Print and shaded views of the part. All mm, measured from the part's lowest x, y and z. A direction names the side the tool comes from. Round coordinates to 2 decimals unless told otherwise and drop trailing zeros. Loops run counter-clockwise (first coordinate to the right, second up) from the corner with the lowest first, then second, coordinate; pieces in that order, holes last. Notation, with made-up numbers: (13, 18) -> (48, 18) arc R25 ccw to (48, 46) -> close; hole circle Ø4 at (-5, -24.75). An arc over 180 degrees is marked (long way). Use a Markdown table: item, result.
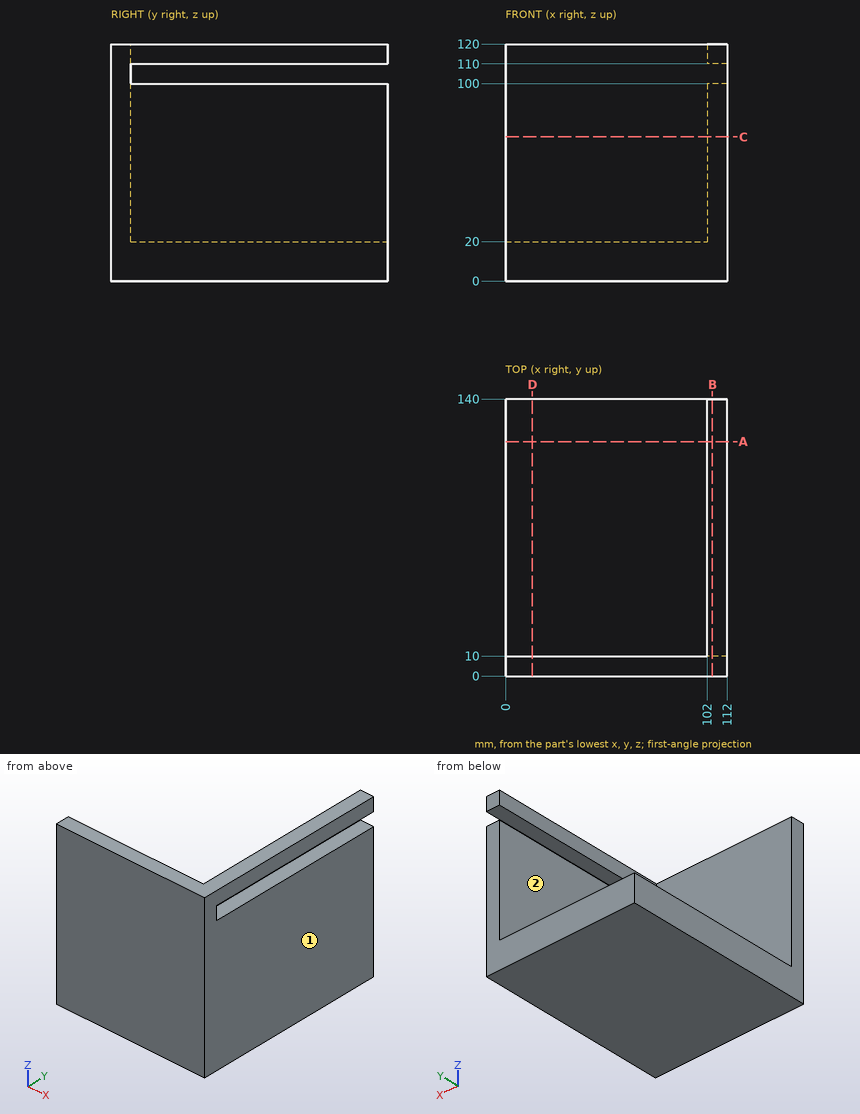
Q1. Tool access for the marked faces 1 and 2: list every direction of +Z, -Z, +X, -X, +Y, -Y with a clear straight run to the whole face (end or side of a thin tool).
Results list:
| item | result |
|---|---|
| face 1 | +Z, -Z, +X, +Y, -Y |
| face 2 | +Z, -X, +Y |
Q2. Flat gauge pins, fed straight in: pin 1 (5 mm diameter, centred on x = 85.5, z = 106, fed in from -Y); pin 2 (2 mm diameter, centred on x = 18, y = 107.5, fed in from +Z); pin 3 (10 mm diameter, centred on x = 65.5, z = 36.5, fed in from +Y); pin 4 (4 mm diameter, centred on y = 110, z = 41, fed in from -X). Where does each tip first touch, or does it go through?
Results list:
| item | result |
|---|---|
| pin 1 | stops at y = 0 |
| pin 2 | stops at z = 20 |
| pin 3 | stops at y = 10 |
| pin 4 | stops at x = 102 |
Q3. Band-saw the part on C-C, the plane z = 73. Give the cut face in (x, y).
Results list:
| item | result |
|---|---|
| outline | (0, 0) -> (112, 0) -> (112, 140) -> (102, 140) -> (102, 10) -> (0, 10) -> close |
Q4. Band-saw the part on A-A, the plane y = 118.5. Give the cut face in (x, z), plus the area to 3 significant figures.
Results list:
| item | result |
|---|---|
| outline | (0, 0) -> (112, 0) -> (112, 100) -> (102, 100) -> (102, 20) -> (0, 20) -> close; (102, 110) -> (112, 110) -> (112, 120) -> (102, 120) -> close |
| area | 3,140 mm² |
Q5. Band-saw the part on B-B, the plane x = 104.5. Give the cut face in (y, z).
Results list:
| item | result |
|---|---|
| outline | (0, 0) -> (140, 0) -> (140, 100) -> (10, 100) -> (10, 110) -> (140, 110) -> (140, 120) -> (0, 120) -> close |
Q6. Band-saw the part on D-D, the plane x = 13.5. Give the cut face in (y, z).
Results list:
| item | result |
|---|---|
| outline | (0, 0) -> (140, 0) -> (140, 20) -> (10, 20) -> (10, 120) -> (0, 120) -> close |
Q7. Drill centre lines: L1, parallel to Z at x = 64, y = 52.5; L2, parallel to X at y = 72.5, z = 90.5; L3, parallel to Y at x = 95, z = 38.5. Where is each one in solid material? Low to high. Write a range as from..to.
Results list:
| item | result |
|---|---|
| L1 | z = 0..20 |
| L2 | x = 102..112 |
| L3 | y = 0..10 |
